The listing builds one solid part. Answer for the finished solid, in the listing's coordinates (mm). A direction names the side the tool comes from. Give positions to 0.01 mm unless a question says otherwise; leave off trailing zeros. Order: outer loops, then holes, each group sorted by start corner. A loop starts at its lowest first (then second) coordinate and runs counter-clockwise, first axis right, second up. Notation, with made-up numbers: (-6.5, -3) - (14.5, -3) arc R14 ccw to (14.5, 3) - close; hole circle Ø11 at (44, 79). An arc over 180 degrees is marked (long way). Answer as a JSON object with one key per item and string values. Group by question number.
Q1. The mould has two halves that part along X. Classify faces 3 (the face through (-72, -70, 1.588)), 4 (the face through (-114.434, 99.74, 0.022)), 5 (the face through (96.55, 94.62, 0.02)): released by +X, released by -X, zero draft, split by the parting line, or undercut.
Q2. For faces 1 (the face through (-107.59, -52.26, 0.02)), 2 (the face through (-91.359, -43.705, 0.022)), determine the directions among +Z, -Z, +X, -X, +Y, -Y from which every point of the face is accessible in a straight line to the end or side of a thin tool.
Q3. Consider line 1 (Y direction, x = 0, z = -0.1); line 2 (X direction, y = 102, z = -1.4); line 3 (X direction, y = 99.5, z = 1.1). Determine where each line is inside the solid, lowest interval first.
Q4. A cutting plane is placed at A-A, the plane x = -106. Give the vertices of the cut face in (y, z).
Q5. Given pin 1 (1 mm diameter, centred on y = -81, z = 0.5, fed in from -X); pin 2 (1.5 mm diameter, centred on y = -41.5, z = 0.5, fed in from +X); pin 3 (0.8 mm diameter, centred on y = -71, z = -0.5, fed in from +X), each flat-ended and moving along its own axis, determine where each tip first touches the part or whether it passes through.
Q6. A cutting plane is placed at C-C, the plane y = 81. Give the vertices of the cut face in (x, z), and give its area (3 significant figures).
Q7. A cutting plane is placed at B-B, the plane z = -0.4. Give the vertices of the cut face in (x, y).
from build123d import *

# Parameters (mm, degrees)
BOSS_EXTRUDE1_DEPTH = 1.5875
CUT_EXTRUDE1_DEPTH  = 3.175
FILLET1_R           = 8.89
CUT_EXTRUDE2_DEPTH  = 212.803448039


with BuildPart() as part:
    # Sketch1 → Boss-Extrude1 (new, symmetric)
    with BuildSketch(Plane.XY):
        with BuildLine():
            Line((-127.293308919, -32.555250036), (-85.984130762, -73.864428193))
            Line((-85.984130762, -73.864428193), (-85.984130762, -86.643760402))
            ThreePointArc((-85.984130762, -86.643760402), (-70.818680903, -97.099597285), (-54.399250036, -105.449308919))
            ThreePointArc((-54.399250036, -105.449308919), (97.88479172, 119.72879172), (-127.293308919, -32.555250036))
        make_face()
    extrude(amount=BOSS_EXTRUDE1_DEPTH, both=True)

    # Sketch2 → Cut-Extrude1 (cut)
    with BuildSketch(Plane.XY.offset(1.5875)):
        with BuildLine():
            Line((-112.423113331, -22.63993873), (-68.458130762, -66.604921299))
            Line((-68.458130762, -66.604921299), (-68.458130762, -77.811715082))
            ThreePointArc((-68.458130762, -77.811715082), (94.55415032, 97.191792757), (-112.423113331, -22.63993873))
        make_face()
    extrude(amount=-CUT_EXTRUDE1_DEPTH, mode=Mode.SUBTRACT)

    # Fillet1
    fillet1_edges = [part.edges().sort_by_distance(p)[0] for p in [
        (-112.423113331, -22.63993873, 0),
        (-68.458130762, -77.811715082, 0),
        (-68.458130762, -66.604921299, 0),
        (-85.984130762, -86.643760402, -0.79375),
        (-85.984130762, -73.864428193, -0.79375),
        (-127.293308919, -32.555250036, -0.79375),
    ]]
    fillet(fillet1_edges, radius=FILLET1_R)

    # Sketch3 → Cut-Extrude2 (cut, through all)
    with BuildSketch(Plane.XY.offset(1.5875)):
        with BuildLine():
            Line((-1.653853322, 152.644117868), (-1.654046603, 160.264117865))
            ThreePointArc((-1.654046603, 160.264117865), (-0.003046821, 160.273999966), (1.647953396, 160.264201621))
            Line((1.647953396, 160.264201621), (1.648146677, 152.644201623))
            Line((1.648146677, 152.644201623), (-1.653853322, 152.644117868))
        make_face()
    extrude(amount=-CUT_EXTRUDE2_DEPTH, mode=Mode.SUBTRACT)


with BuildPart() as cut_extrude2_kept_piece:
    # of the separate pieces the step leaves, the one the design keeps (cut_extrude2_pieces_kept)
    add(part.part.solids().sort_by_distance((-126.058425896, -33.790133059, -1.5875))[0])


solid = cut_extrude2_kept_piece.part
Reply:
{
 "1": {"face 3": "zero draft", "face 4": "released by -X", "face 5": "undercut"},
 "2": {"face 1": "+Z, -Z, -X, -Y", "face 2": "+Z, -Z"},
 "3": {"line 1": "y = -116.59 to -99.06, 142.75 to 152.64", "line 2": "x = -112.86 to -90.51, 90.51 to 112.86", "line 3": "x = -114.6 to -92.67, 92.67 to 114.6"},
 "4": {"outline": "(-53.85, -1.59) - (-29.06, -1.59) - (-29.06, 1.59) - (-53.85, 1.59) - close; (80, -1.59) - (110.88, -1.59) - (110.88, 1.59) - (80, 1.59) - close"},
 "5": {"pin 1": "stops at x = -85.98", "pin 2": "stops at x = 123.47", "pin 3": "stops at x = 103.04"},
 "6": {"outline": "(-125.15, -1.59) - (-105.44, -1.59) - (-105.44, 1.59) - (-125.15, 1.59) - close; (105.44, -1.59) - (125.15, -1.59) - (125.15, 1.59) - (105.44, 1.59) - close", "area": "125 mm^2"},
 "7": {"outline": "(-127.99, -30.89) arc R8.89 ccw to (-126.06, -33.79) - (-88.59, -71.26) arc R8.89 cw to (-85.98, -77.55) - (-85.98, -82.26) arc R8.89 ccw to (-82.38, -89.4) arc R138.43 ccw (long way) to (1.65, 160.26) - (1.65, 152.64) - (-1.65, 152.64) - (-1.65, 160.26) arc R138.43 ccw to start; hole (-113.13, -20.82) arc R8.89 ccw to (-111.09, -23.97) - (-71.06, -64) arc R8.89 cw to (-68.46, -70.29) - (-68.46, -73.02) arc R8.89 ccw to (-64.3, -80.55) arc R120.9 ccw (long way) to start"}
}
